from build123d import *

# Parameters (mm, degrees)
F1_DEPTH = 16
F2_W     = 70
F2_H     = 2
F2_H_2   = 10
F3_DEPTH = 2
F4_R     = 1


with BuildPart() as f1:
    # F0 (on Front) → F1 (new body)
    with BuildSketch(Plane.XZ):
        with BuildLine():
            ThreePointArc((0, -9), (-9, 0), (0, 9))
            Line((0, 9), (74, 9))
            Line((74, 9), (74, 11))
            Line((74, 11), (0, 11))
            ThreePointArc((0, 11), (-11, 0), (0, -11))
            Line((0, -11), (18.2864816057, -11))
            ThreePointArc((18.2864816057, -11), (20.6021054823, -11.7384227646), (22.0627746665, -13.6810569689))
            ThreePointArc((22.0627746665, -13.6810569689), (39.0966080524, -40.824002055), (66.2209606463, -57.8874262169))
            ThreePointArc((66.2209606463, -57.8874262169), (69.6378774832, -59.6435957626), (72.4487811093, -62.2624262169))
            Line((72.4487811093, -62.2624262169), (74, -61))
            ThreePointArc((74, -61), (70.7875387131, -58.0070509094), (66.8824908995, -56))
            ThreePointArc((66.8824908995, -56), (40.2783781222, -39.1759850939), (23.7357366507, -12.396005494))
            ThreePointArc((23.7357366507, -12.396005494), (21.9137628138, -9.9367517594), (19, -9))
            Line((19, -9), (0, -9))
        make_face()
    extrude(amount=F1_DEPTH)

    # F2 (on face) → F3 (join)
    with BuildSketch(Plane.XZ.offset(16)):
        with Locations((39, 10)):
            Rectangle(F2_W, F2_H)
        with Locations((39, 4)):
            Rectangle(F2_W, F2_H_2)
    extrude(amount=F3_DEPTH)

    # F4
    f4_edges = [f1.edges().sort_by_distance(p)[0] for p in [
        (39, -18, 11),
        (39, -16, 9),
    ]]
    fillet(f4_edges, radius=F4_R)

    # F5: F1 across plane


with BuildPart() as f1_1:
    add(f1.part)
    add(f1.part.mirror(Plane.XZ))


solid = f1_1.part
Part model, mm, in its own coordinate system. A direction names the side the tool comes from. Round coordinates to 2 decimals unless told otherwise and drop trailing zeros. Order: outer loops, then holes, each group sorted by start corner. A loop starts at its lowest first (then second) coordinate and runs counter-clockwise, first axis right, second up. Notation, with made-up numbers: (86.5, -35.5) -> (115.5, -35.5) arc R29 cw to (115.5, -9.5) -> close; hole circle Ø4 at (-29.75, 30.5). An arc over 180 degrees is marked (long way). Put each result on its own line as item: value.
Q1. Wall check: line 1 (Y direction, x = 52, z = 0); line 2 (Z direction, x = 10.5, y = -8.5); line 3 (Z direction, x = 65, y = 13). Give the ranges that are in metal, low to high. Write a range as [from, to].
From the geometry:
line 1: y = [-18, -16], [16, 18]
line 2: z = [-11, -9], [9, 11]
line 3: z = [-57.45, -55.31], [9, 11]
Q2. Tool access for faces 4 (the face through (25, 16, -20)), 5 (the face through (39, -16, 4)), 6 (the face through (25, -16, -20)), 7 (the face through (10, 0, -9)), 8 (the face through (39, -17, -1)): list every direction of +Z, -Z, +X, -X, +Y, -Y with a clear straight run to the whole face (end or side of a thin tool).
From the geometry:
face 4: -Z, -X, +Y
face 5: +X
face 6: -Z, -X, -Y
face 7: +X, +Y, -Y
face 8: -Z, +X, -X, +Y, -Y
Q3. Pin check, flat tips, straight feed: pin 1 Ø5 at (y, z) = (-1, -54.5) entering from +X; pin 2 Ø14.5 at (x, y) = (8, -6.5) entering from -Z; pin 3 Ø1.5 at (y, z) = (-16.5, 4.5) entering from -X; pin 4 Ø10 at (x, z) = (62, -6.5) entering from -Y. Stop position of each tip, or through.
From the geometry:
pin 1: stops at x = 69.15
pin 2: stops at z = -11
pin 3: stops at x = -10.27
pin 4: passes through
Q4. Band-saw the part on B-B (x = 2). Give the cut face in (y, z), and give its area (3 significant figures).
From the geometry:
outline: (-16, -11) -> (16, -11) -> (16, -9) -> (-16, -9) -> close; (-16, 9) -> (16, 9) -> (16, 11) -> (-16, 11) -> close
area: 128 mm2
Q5. Pull direction Z, two halves, no side cores. Call faces 1 (the face through (22, 0, -10)), 2 (the face through (74, -2.8, 9.4)), 3 (the face through (9, 0, -11)): pulls with the +Z half, pulls with the -Z half, needs draft (parallel to the pull), parting line crosses it, or undercut.
From the geometry:
face 1: undercut
face 2: needs draft
face 3: pulls with the -Z half
Q6. Band-saw the part on C-C (y = 8). Give the cut face in (x, z), and give its area (3 significant figures).
From the geometry:
outline: (0, -11) -> (18.29, -11) arc R4 cw to (22.06, -13.68) arc R72 ccw to (66.22, -57.89) arc R14 cw to (72.45, -62.26) -> (74, -61) arc R16 ccw to (66.88, -56) arc R70 cw to (23.74, -12.4) arc R5 ccw to (19, -9) -> (0, -9) arc R9 cw to (0, 9) -> (74, 9) -> (74, 11) -> (0, 11) arc R11 ccw to start
area: 405 mm2
Q7. Band-saw the part on A-A (z = 0). Give the cut face in (x, y).
From the geometry:
outline: (-11, -16) -> (-9, -16) -> (-9, 16) -> (-11, 16) -> close; (4, -18) -> (74, -18) -> (74, -16) -> (4, -16) -> close; (4, 16) -> (74, 16) -> (74, 18) -> (4, 18) -> close
Q8. Band-saw the part on D-D (x = 54). Give the cut face in (y, z).
From the geometry:
outline: (-18, -1) -> (-16, -1) -> (-16, 8) arc R1 cw to (-15, 9) -> (15, 9) arc R1 cw to (16, 8) -> (16, -1) -> (18, -1) -> (18, 10) arc R1 ccw to (17, 11) -> (-17, 11) arc R1 ccw to (-18, 10) -> close; (-16, -52.27) -> (16, -52.27) -> (16, -49.95) -> (-16, -49.95) -> close
